Geometry: final body of the model. Coordinates: model frame, mm. Give positions to 0.01 mm unless a question says otherwise; leave off trailing zeros. Order: outer loops, then holes, each group sorted by start corner. A loop starts at its lowest first (then second) coordinate and runs counter-clockwise, first axis right, second up. Notation, with made-up numbers: (57, -30) - (112, -30) arc R34 cw to (112, 1) - close; hole circle Ø3 at (56, 46.5). An arc over 180 degrees is marked (long way). One line per item, written item: value.
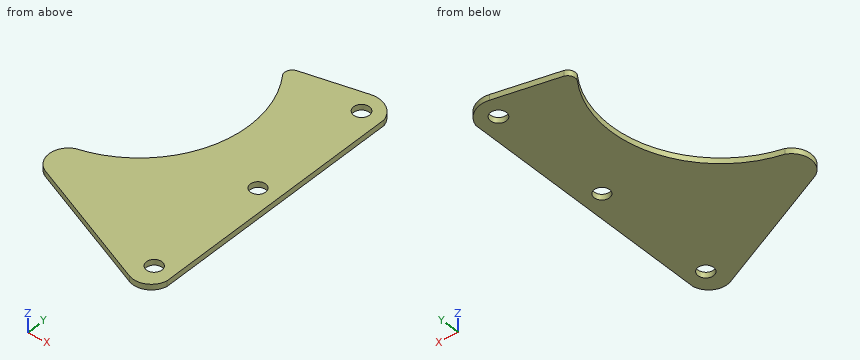
```python
from build123d import *

# Parameters (mm, degrees)
F0_R     = 2.492008
F0_R_2   = 2.45277
F0_R_3   = 2.539594
F1_DEPTH = 1.8


with BuildPart() as f1:
    # F0 (on Top) → F1 (new body)
    with BuildSketch(Plane.XY):
        with BuildLine():
            Line((-50.339356, -66.981845), (-8.10042, -84.58598))
            ThreePointArc((-8.10042, -84.58598), (-2.989306, -84.200884), (0, -80.037251))
            Line((0, -80.037251), (0, 1.829881))
            ThreePointArc((0, 1.829881), (-3.406029, 6.28153), (-8.948847, 7.11543))
            Line((-8.948847, 7.11543), (-28.766483, 2.37366))
            ThreePointArc((-28.766483, 2.37366), (-30.224163, 1.08954), (-30.308826, -0.851239))
            ThreePointArc((-30.308826, -0.851239), (-25.761186, -33.597985), (-50.339356, -55.710062))
            ThreePointArc((-50.339356, -55.710062), (-53.87346, -61.345953), (-50.339356, -66.981845))
        make_face()
        with Locations((-6.138234, -77.649219)):
            Circle(F0_R, mode=Mode.SUBTRACT)
        with Locations((-6.351363, -38.250507)):
            Circle(F0_R_2, mode=Mode.SUBTRACT)
        with Locations((-6.43489, 0.851118)):
            Circle(F0_R_3, mode=Mode.SUBTRACT)
    extrude(amount=F1_DEPTH)


solid = f1.part
```
1) Section A-A, the plane x = -7. Return loops of the section in (y, z), then the cut area to 3 significant figures.
Answers below:
outline: (-84.89, 0) - (-79.99, 0) - (-79.99, 1.8) - (-84.89, 1.8) - close; (-75.31, 0) - (-40.62, 0) - (-40.62, 1.8) - (-75.31, 1.8) - close; (-35.89, 0) - (-1.62, 0) - (-1.62, 1.8) - (-35.89, 1.8) - close; (3.33, 0) - (7.32, 0) - (7.32, 1.8) - (3.33, 1.8) - close
area: 140 mm^2
2) Section B-B, the plane z = 1.2. Return loops of the section in (x, y), then the cut area to 3 significant figures.
Answers below:
outline: (-50.34, -66.98) - (-8.1, -84.59) arc R6.06 ccw to (0, -80.04) - (0, 1.83) arc R7.48 ccw to (-8.95, 7.12) - (-28.77, 2.37) arc R2.48 ccw to (-30.31, -0.85) arc R35.25 cw to (-50.34, -55.71) arc R6.26 ccw to start; hole circle Ø5.08 at (-6.43, 0.85); hole circle Ø4.91 at (-6.35, -38.25); hole circle Ø4.98 at (-6.14, -77.65)
area: 2,800 mm^2
3) Material intervals for line 1 along Y through (x, z) = (-5, 0.5); line 2 along Y through (x, z) = (-29, 0.9); line 3 along Y through (x, z) = (-27, 0.25), sorted ascending.
Answers below:
line 1: -84.9 to -79.87, -75.43 to -40.3, -36.2 to -1.24, 2.95 to 6.99
line 2: -75.88 to -40.22, -2.79 to 2.28
line 3: -76.71 to -36.56, -6.45 to 2.8
4) Section D-D, the plane y = -18. Return loops of the section in (x, z), then the cut area to 3 significant figures.
Answers below:
outline: (-23.8, 0) - (0, 0) - (0, 1.8) - (-23.8, 1.8) - close
area: 42.8 mm^2
5) First-contact query: pin 1 (5.5 mm diameter, centred on x = -6.35, y = -38.25, fed in from -Z); pin 2 (3 mm diameter, centred on x = -6.14, y = -77.65, fed in from +Z). Flat tips, straight axial feed; report the tip coordinate or a pass-through.
Answers below:
pin 1: z = 0
pin 2: through
6) Section C-C, the plane y = -76.5. Return loops of the section in (x, z), then the cut area to 3 significant figures.
Answers below:
outline: (-27.5, 0) - (-8.35, 0) - (-8.35, 1.8) - (-27.5, 1.8) - close; (-3.93, 0) - (0, 0) - (0, 1.8) - (-3.93, 1.8) - close
area: 41.5 mm^2
